Autodesk Fusion 360 part; units mm, degrees
sketch "Sketch2" plane through (0, 1.6535, 0) normal (0, 1, 0) x (-1, 0, 0)
  line L0 (-63.6703, 1) -> (-5.6703, 1)
  line L1 (-5.6703, 1) -> (-5.6703, 7)
  line L2 (-5.6703, 7) -> (-63.6703, 7)
  line L3 (-63.6703, 7) -> (-63.6703, 1)
  line L4 (-30.5955, 7) -> (-38.4299, 7)
  line L5 (-38.4299, 7) -> (-38.4299, 2)
  line L6 (-38.4299, 2) -> (-30.5955, 2)
  line L7 (-30.5955, 2) -> (-30.5955, 7)
  dimension "d1" = 5
sketch "Sketch3" plane through (0, 0, 1) normal (0, 0, 1) x (1, 0, 0)
  circle A0 centre (9.6172, 60.4797) radius 2.5
  circle A1 centre (60.4172, 9.6797) radius 2.5
  circle A2 centre (9.6172, 9.6797) radius 2.5
  circle A3 centre (60.4172, 60.4797) radius 2.5
  line L0 (68.4203, 4.9035) -> (68.4203, 64.4035)
  arc A4 (68.4203, 64.4035) -> (64.4203, 68.4035) centre (64.4203, 64.4035) ccw
  line L1 (64.4203, 68.4035) -> (4.9203, 68.4035)
  arc A5 (4.9203, 68.4035) -> (0.9203, 64.4035) centre (4.9203, 64.4035) ccw
  line L2 (0.9203, 64.4035) -> (0.9203, 4.9035)
  arc A6 (0.9203, 4.9035) -> (4.9203, 0.9035) centre (4.9203, 4.9035) ccw
  line L3 (4.9203, 0.9035) -> (64.4203, 0.9035)
  arc A7 (64.4203, 0.9035) -> (68.4203, 4.9035) centre (64.4203, 4.9035) ccw
  line L4 (5.6703, 67.6535) -> (63.6703, 67.6535)
  line L5 (67.6703, 63.6535) -> (67.6703, 5.6535)
  line L6 (63.6703, 1.6535) -> (5.6703, 1.6535)
  line L7 (1.6703, 5.6535) -> (1.6703, 63.6535)
  arc A8 (5.6703, 67.6535) -> (1.6703, 63.6535) centre (5.6703, 63.6535) ccw
  arc A9 (67.6703, 63.6535) -> (63.6703, 67.6535) centre (63.6703, 63.6535) ccw
  arc A10 (63.6703, 1.6535) -> (67.6703, 5.6535) centre (63.6703, 5.6535) ccw
  arc A11 (1.6703, 5.6535) -> (5.6703, 1.6535) centre (5.6703, 5.6535) ccw
  dimension "d2" = 4
  dimension "d3" = 0.75
  dimension "d4" = 0.75
  dimension "d5" = 0.75
  dimension "d6" = 0.75
sketch "Sketch1" plane through (0, 0, 0) normal (0, 0, 1) x (1, 0, 0)
  circle A0 centre (9.6172, 9.6797) radius 1.5
  circle A1 centre (60.4172, 9.6797) radius 1.5
  arc A2 (4.9203, 69.4035) -> (-0.0797, 64.4035) centre (4.9203, 64.4035) ccw
  arc A3 (64.4203, -0.0965) -> (69.4203, 4.9035) centre (64.4203, 4.9035) ccw
  circle A4 centre (60.4172, 60.4797) radius 1.5
  line L0 (-6, 9.6797) -> (72, 9.6797) construction
  line L1 (35.0172, 92) -> (35.0172, -8) construction
  line L2 (64.4203, 69.4035) -> (4.9203, 69.4035)
  line L3 (60.4172, -4) -> (60.4172, 71) construction
  line L4 (-7, 60.4797) -> (90.0735, 60.4797) construction
  arc A5 (69.4203, 64.4035) -> (64.4203, 69.4035) centre (64.4203, 64.4035) ccw
  line L5 (4.9203, -0.0965) -> (64.4203, -0.0965)
  line L6 (-7, 66.8297) -> (83, 66.8297) construction
  arc A6 (-0.0797, 4.9035) -> (4.9203, -0.0965) centre (4.9203, 4.9035) ccw
  line L7 (-0.0797, 64.4035) -> (-0.0797, 4.9035)
  line L8 (-5, 3.3297) -> (86.8002, 3.3297) construction
  line L9 (9.6172, 82) -> (9.6172, -14) construction
  line L10 (69.4203, 4.9035) -> (69.4203, 64.4035)
  circle A7 centre (9.6172, 60.4797) radius 1.5
  point P0 (2.2672, 67.8297)
  point P1 (67.7672, 67.8297)
  point P2 (69.4203, -0.0965)
  point P3 (69.4203, 69.4035)
  point P4 (-0.0797, 69.4035)
  dimension "d138" = 69.5
  dimension "d139" = 69.5
  dimension "d140" = 65.5
  dimension "d143" = 6.35
  dimension "d144" = 6.35
  dimension "d156" = 3
  dimension "d158" = 3
  dimension "d160" = 3
  dimension "d162" = 3
  dimension "d164" = 5
  dimension "d165" = 5
  dimension "d166" = 5
  dimension "d167" = 5
extrude "Extrude1" add sketch "Sketch1" along normal blind 5
shell "Shell1" thickness 1 removed faces 1 at (26.9171, 26.9532, 5)
extrude "Extrude3" add sketch "Sketch3" along normal blind 6 contours L0 A4 L1 A5 L2 A6 L3 A7
hole "Hole2" at (60.4172, 60.4797, 0) direction (0, 0, 1) diameter 3 depth 3 tip angle 118 countersink diameter 7 countersink angle 120
hole "Hole10" at (60.4172, 9.6797, 0) direction (0, 0, 1) diameter 3 depth 2.75 tip angle 118 countersink diameter 7 countersink angle 120
hole "Hole11" at (9.6172, 9.6797, 0) direction (0, 0, 1) diameter 3 depth 2.75 tip angle 118 countersink diameter 7 countersink angle 120
hole "Hole12" at (9.6172, 60.4797, 0) direction (0, 0, 1) diameter 3 depth 2.75 tip angle 118 countersink diameter 7 countersink angle 120
extrude "Extrude4" cut sketch "Sketch2" against normal blind 2 contours L2 L4 L5 L6 L7
equation "d143 = mount_post_offset"
equation "d144 = mount_post_offset"
equation "d156 = mount_post_pcb_holder"
equation "d158 = mount_post_pcb_holder"
equation "d160 = mount_post_pcb_holder"
equation "d162 = mount_post_pcb_holder"
equation "d164 = shell_corner_radius"
equation "d165 = shell_corner_radius"
equation "d166 = shell_corner_radius"
equation "d167 = shell_corner_radius"
equation "mount_post_offset = 6.35 mm"
equation "mount_post_pcb_holder = 3 mm"
equation "shell_corner_radius = 5 mm"
Could you check a few things on this model? Use its own coordinates, in mm. A direction names the side the tool comes from. Give positions to 0.01 mm unless a question says otherwise; leave off trailing zeros. Loops run counter-clockwise (first coordinate to the right, second up) from the corner with the lowest first, then second, coordinate; pieces in that order, holes last. Notation, with made-up numbers: (67.25, 77.5) -> (103.25, 77.5) arc R19 ccw to (103.25, 81.5) -> close; hole circle Ø11 at (88.25, 73.5). An arc over 180 degrees is marked (long way). Put each result on its own line as item: value.
(1) Thinking about a two-plate mould opening in Y: for faces 4 (the face through (34, 35, 0)), 5 (the face through (35, 68.404, 6)), 6 (the face through (57.92, 9.57, 2.97)), which applies, pulls with the +Y half, pulls with the -Y half, needs draft (parallel to the pull), parting line crosses it, or undercut?
Computed:
face 4: needs draft
face 5: pulls with the +Y half
face 6: undercut
(2) For faces 1 (the face through (30.596, 1, 4)), 2 (the face through (60.4, 58.8, 5)), 3 (the face through (1.424, 1.329, 2.465)), which set-ups out of +Z, -Z, +X, -X, +Y, -Y let a thin tool reach every point of the face, with its end or its side?
Computed:
face 1: +Z, -Y
face 2: +Z
face 3: +Z, -Z, -X, -Y
(3) I'm going to push flat-ended pins straight in: pin 1 Ø2.5 at (x, y) = (10.5, 61.5) entering from +Z; pin 2 Ø2.5 at (x, y) = (9.62, 9.68) entering from -Z; pin 3 Ø1.9 at (y, z) = (1, 5.5) entering from +X; pin 4 Ø0.6 at (x, z) = (14.5, 6) entering from -Y. Where does each tip first touch, or does it pass through?
Computed:
pin 1: z = 5
pin 2: through
pin 3: x = 68.35
pin 4: y = 0.9
(4) Imagine slicing it at A-A on y = 28. Write out the boundary of the cut face in (x, z), plus the area to 3 significant figures.
Computed:
outline: (-0.08, 0) -> (69.42, 0) -> (69.42, 5) -> (68.42, 5) -> (68.42, 7) -> (67.67, 7) -> (67.67, 1) -> (1.67, 1) -> (1.67, 7) -> (0.92, 7) -> (0.92, 5) -> (-0.08, 5) -> close
area: 86.5 mm^2
(5) Imagine slicing it at B-B on x = 15.5. Write out the boundary of the cut face in (y, z), plus the area to 3 significant figures.
Computed:
outline: (-0.1, 0) -> (69.4, 0) -> (69.4, 5) -> (68.4, 5) -> (68.4, 7) -> (67.65, 7) -> (67.65, 1) -> (1.65, 1) -> (1.65, 7) -> (0.9, 7) -> (0.9, 5) -> (-0.1, 5) -> close
area: 86.5 mm^2
(6) Please list where these lines run through material, in increasing order: probe 1 along X at (y, z) = (60.5, 2.25); probe 2 along X at (y, z) = (54, 5.5); probe 3 along Y at (x, z) = (15, 2.75). Write a range as [from, to].
Computed:
probe 1: [-0.08, 1.67], [7.12, 8.12], [11.12, 12.12], [57.92, 58.92], [61.92, 62.92], [67.67, 69.42]
probe 2: [0.92, 1.67], [67.67, 68.42]
probe 3: [-0.1, 1.65], [67.65, 69.4]
